Here's the drawing with two shaded views (mm, measured from the low corner). I have some questions. Round coordinates to 2 decimals unless told otherwise and drop trailing zeros. Order: outer loops, then holes, each group sorted by start corner. A loop starts at its lowest first (then second) coordinate and runs counter-clockwise, first axis right, second up. Notation, with made-up numbers: (79, -38.5) -> (85, -38.5) arc R18 cw to (85, -32.5) -> close; hole circle Ø4 at (-2, 55.5). An arc over 180 degrees is marked (long way). Put each result on its own line as item: value. Start each with the question number.
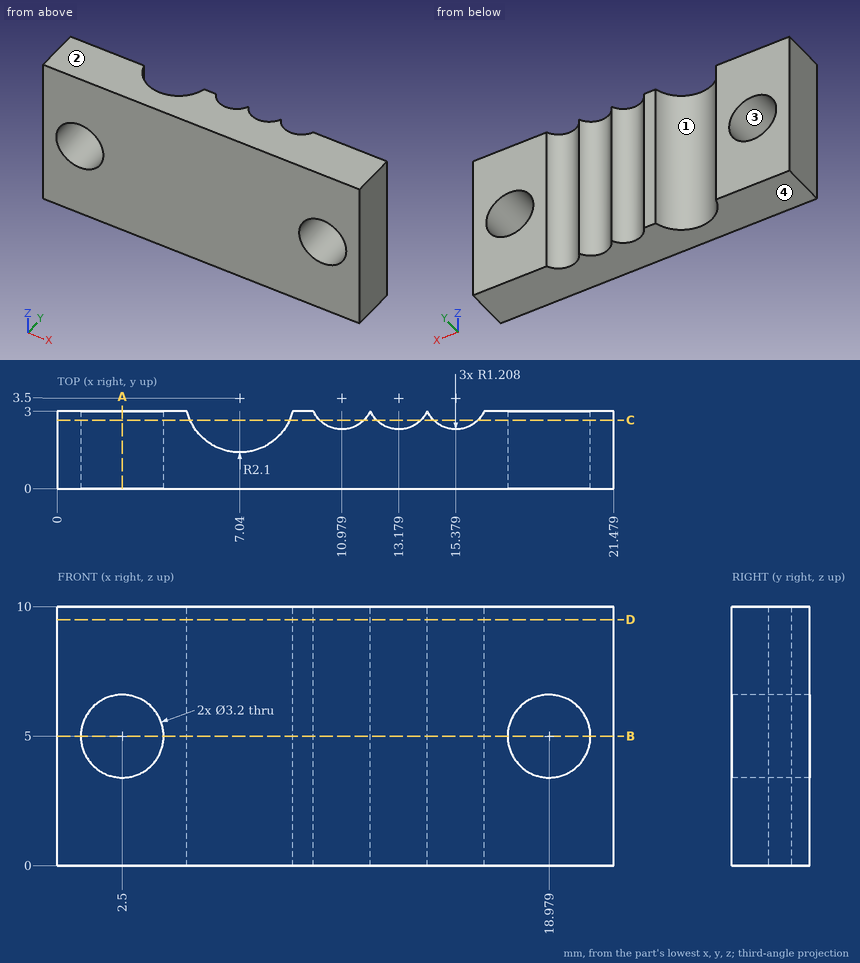
1. If we section it at D-D, the plane z = 9.5: Please give me the cut outline in (x, y).
2. I need wall thicknesses on L1, parallel to X at y = 2.55, z = 8.75 (1 decimal); L2, parallel to Z at x = 2.5, y = 0.75; L3, parallel to X at y = 0.7, z = 4.5. Which ranges of each line are inside material? Lowest first, please.
3. If we section it at B-B, the plane z = 5: Please give me the cut outline in (x, y).
4. Thinking about a two-plate mould opening in Z: for the marked faces 1, 2, 3 and 4, which applies, +Z half, -Z half, draft (parallel to the pull), parting line (faces both ways), or undercut?
5. If we section it at A-A, the plane x = 2.5: Please give me the cut outline in (y, z), then the cut area to 3 significant figures.
6. If we section it at C-C, the plane y = 2.65: Please give me the cut outline in (x, z), then the cut area to 3 significant figures.
Results below:
1. outline: (0, 0) -> (21.48, 0) -> (21.48, 3) -> (16.48, 3) arc R1.21 cw to (14.28, 3) arc R1.21 cw to (12.08, 3) arc R1.21 cw to (9.88, 3) -> (9.08, 3) arc R2.1 cw to (5, 3) -> (0, 3) -> close
2. L1: 0 to 5.2, 8.9 to 10.2, 11.7 to 12.4, 13.9 to 14.6, 16.1 to 21.5
2. L2: 0 to 3.4, 6.6 to 10
2. L3: 0 to 0.98, 4.02 to 17.46, 20.5 to 21.48
3. outline: (0, 0) -> (0.9, 0) -> (0.9, 3) -> (0, 3) -> close; (4.1, 0) -> (17.38, 0) -> (17.38, 3) -> (16.48, 3) arc R1.21 cw to (14.28, 3) arc R1.21 cw to (12.08, 3) arc R1.21 cw to (9.88, 3) -> (9.08, 3) arc R2.1 cw to (5, 3) -> (4.1, 3) -> close; (20.58, 0) -> (21.48, 0) -> (21.48, 3) -> (20.58, 3) -> close
4. face 1: draft
4. face 2: +Z half
4. face 3: undercut
4. face 4: -Z half
5. outline: (0, 0) -> (3, 0) -> (3, 3.4) -> (0, 3.4) -> close; (0, 6.6) -> (3, 6.6) -> (3, 10) -> (0, 10) -> close
5. area: 20.4 mm2
6. outline: (0, 0) -> (5.12, 0) -> (5.12, 10) -> (0, 10) -> close; (8.96, 0) -> (10.12, 0) -> (10.12, 10) -> (8.96, 10) -> close; (11.84, 0) -> (12.32, 0) -> (12.32, 10) -> (11.84, 10) -> close; (14.04, 0) -> (14.52, 0) -> (14.52, 10) -> (14.04, 10) -> close; (16.24, 0) -> (21.48, 0) -> (21.48, 10) -> (16.24, 10) -> close; hole circle Ø3.2 at (2.5, 5); hole circle Ø3.2 at (18.98, 5)
6. area: 109 mm2
